Geometry check sheet. Reference: drawing and pictorial views, mm from the part's lowest x, y, z. A direction names the side the tool comes from. Give positions to 0.01 mm unless a question says otherwise; leave off trailing zeros. Loops run counter-clockwise (first coordinate to the right, second up) from the corner with the lowest first, then second, coordinate; pieces in that order, holes last. Notation, with made-up numbers: (48, -6) -> (107, -6) arc R7 ccw to (107, 0) -> close; hole circle Ø11 at (8.5, 32.5). An arc over 180 degrees is marked (long way). One line per item, written item: value. Start each with the question number.
(1) Sectioned sample at C-C, the plane y = 1.75. Record the cut outline in (x, z).
(2) Scan lines: line 1 along Z through (x, y) = (9, 3.75); line 2 along Y through (x, z) = (5.25, 2). Record each from-to range of solid material in increasing order. Write a range as from..to.
(3) Gauge pin test, flat ends, axial feed: pin 1 Ø5 at (x, y) = (10.5, 5) entering from +Z; pin 2 Ø2 at (y, z) = (2.5, 7) entering from +X; pin 3 Ø3 at (y, z) = (9, 5.5) entering from +X; pin 4 Ø9 at (x, z) = (9, 9) entering from +Y (1 decimal). Record the tip position at first contact, or that the pin passes through.
(4) Tool access check on the marked faces 1 and 2. Record the directions out of +Z, -Z, +X, -X, +Y, -Y that give a thin tool (end or side, any length) a straight path to the whole face; none if there is none.
(5) Sectioned sample at B-B, the plane z = 9. Record the cut outline in (x, y), then the cut area to 3 significant figures.
(6) Sectioned sample at A-A, the plane x = 9. Record the cut outline in (y, z), then the cut area to 3 significant figures.
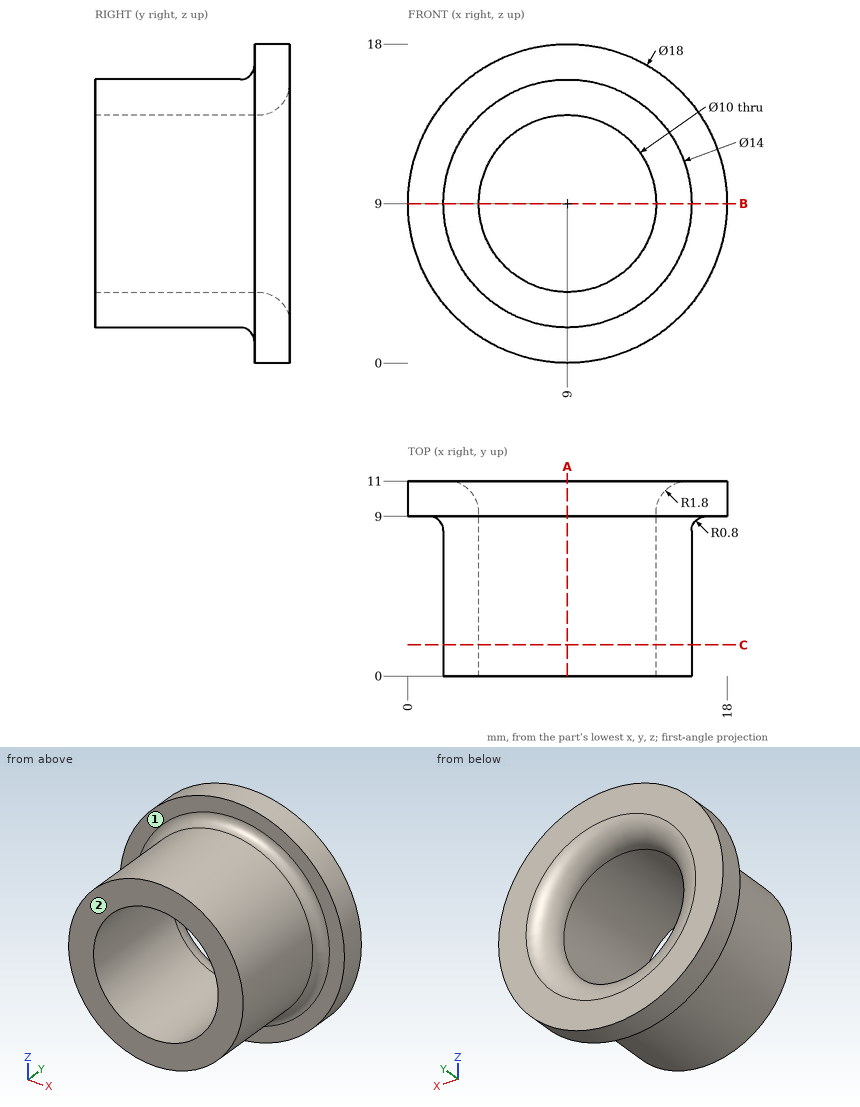
Calculated:
1. outline: circle Ø14 at (9, 9); hole circle Ø10 at (9, 9)
2. line 1: z = 2..4, 14..16
2. line 2: y = 9..11
3. pin 1: stops at z = 16
3. pin 2: stops at x = 15.93
3. pin 3: stops at x = 17.77
3. pin 4: passes through
4. face 1: -Y
4. face 2: +Z, -Z, +X, -X, -Y
5. outline: (0, 9) -> (1.2, 9) arc R0.8 cw to (2, 8.2) -> (2, 0) -> (4, 0) -> (4, 9.2) arc R1.8 ccw to (2.2, 11) -> (0, 11) -> close; (14, 0) -> (16, 0) -> (16, 8.2) arc R0.8 cw to (16.8, 9) -> (18, 9) -> (18, 11) -> (15.8, 11) arc R1.8 ccw to (14, 9.2) -> close
5. area: 50.9 mm2
6. outline: (0, 2) -> (8.2, 2) arc R0.8 cw to (9, 1.2) -> (9, 0) -> (11, 0) -> (11, 2.2) arc R1.8 ccw to (9.2, 4) -> (0, 4) -> close; (0, 14) -> (9.2, 14) arc R1.8 ccw to (11, 15.8) -> (11, 18) -> (9, 18) -> (9, 16.8) arc R0.8 cw to (8.2, 16) -> (0, 16) -> close
6. area: 50.9 mm2
